Autodesk Inventor part; units mm, degrees
ref_plane "YZ Plane" through (0, 0, 0) normal (1, 0, 0) x (0, 1, 0)
ref_plane "XZ Plane" through (0, 0, 0) normal (0, 1, 0) x (-1, 0, 0)
ref_plane "XY Plane" through (0, 0, 0) normal (0, 0, 1) x (1, 0, 0)
sketch "Sketch1" plane through (0, 0, 0) normal (0, 0, 1) x (1, 0, 0)
  line L0 (-22.529, 12.5) -> (-14.529, 12.5)
  line L1 (22.5896, 12.5) -> (14.571, 12.5)
  line L2 (12.171, 14.9) -> (22.5896, 14.9)
  line L3 (22.5896, 14.9) -> (22.5896, 12.5)
  line L4 (-12.129, 14.9) -> (-22.529, 14.9)
  line L5 (-22.529, 14.9) -> (-22.529, 12.5)
  line L6 (-12.129, 0) -> (-12.129, 14.9)
  line L7 (12.171, 0) -> (12.171, 14.9)
  arc A0 (-12.129, 0) -> (12.171, 0) centre (0.021, 0) ccw
  arc A1 (-14.529, 0) -> (14.571, 0) centre (0.021, 0) ccw
  line L8 (-14.529, 12.5) -> (-14.529, -0.0004)
  line L9 (14.571, 12.5) -> (14.571, 0)
  point P0 (0, 0)
  point P1 (14.6524, 0.7379)
  dimension "d34" = 14.9
  dimension "d35" = 14.9
  dimension "d38" = 2.4
  dimension "d39" = 2.4
  dimension "d46" = 24.3
  dimension "d47" = 2.4
  dimension "d48" = 2.4
extrude "Extrusion5" add sketch "Sketch1" along normal blind 6
fillet "Fillet7" radius 1 1 edges at (14.571, 12.5, 3)
fillet "Fillet8" radius 1 1 edges at (-14.529, 12.5, 3)
sketch "Sketch5" plane through (12.171, 14.9, 0) normal (0, 1, 0) x (1, 0, 0)
  line L0 (10.4185, 0) -> (10.4185, -6)
  line L1 (3.4, 0) -> (10.4185, 0)
  circle A0 centre (5.2093, -3) radius 1.5
  circle A1 centre (-29.5299, -3.1217) radius 1.5
  point P0 (-12.171, 0)
  dimension "d54" = 3
extrude "Extrusion6" cut sketch "Sketch5" against normal blind 10
properties part number "motor_support_v2" material "PET Plastic"
For this review, take the finished solid that the model builds, in its own axes (mm). A direction names the side the tool comes from. Give positions to 0.01 mm unless a question says otherwise; leave off trailing zeros. Loops run counter-clockwise (first coordinate to the right, second up) from the corner with the lowest first, then second, coordinate; pieces in that order, holes last. Notation, with made-up numbers: M 12,56.25 L 44,56.25 A28 ccw 44,78.25 Z; hole C -26,-31.75 d4. An arc over 180 degrees is marked long. Answer as a JSON object with one key per item and string values. Group by question number.
Q1. Add section C-C on y = 7. Give the boundary of the cut face in (x, z), and give its area (3 significant figures).
Q2. Add section A-A on y = -9.75. Give the boundary of the cut face in (x, z).
Q3. Mouldability with a two-part tool opening along X and no side actions: class faces 1 (the flat face through (22.59, 14, 3)), 2 (the flat face through (-12, -3, 0)), 3 (the flat face through (12.171, 7, 3)), 4 (the flat face through (-12.129, 7, 3)) as +X half, -X half, draft (parallel to the pull), parting line (faces both ways), or undercut.
Q4. Insertion check: P1, Ø3, axis at y = 4.5, z = 4, coming from the +X side; P2, Ø2.5, axis at x = -17.36, z = 3.12, coming from the +Y side; P3, Ø1.8, axis at x = -19.5, z = 3, coming from the -Y side; P4, Ø3, axis at y = 5, z = 4, coming from the -X side. Each pin has a flat end and moves straight along its axis. Give the tip position at first contact, or say it passes through.
Q5. Tool access review of faces 5 (the flat face through (-19.1, 12.5, 3)), 6 (the flat face through (16, 14.9, 2)), 7 (the flat face through (19.1, 12.5, 3)): name each direction out of +Z, -Z, +X, -X, +Y, -Y from which nothing blocks a thin tool from reaching the whole face with its end or side.
Q6. Add section D-D on x = -4. Give the boundary of the cut face in (y, z).
Q7. Add section B-B on z = 2.45. Give the boundary of the cut face in (x, y), and give its area (3 significant figures).
Q8. For probe 1 along X at (y, z) = (13.55, 3); probe 2 along X at (y, z) = (3.5, 4.4); probe 3 along Y at (x, z) = (17, 4.65), list the stretches that pass through material, from the lowest coordinate up. Write a range as [from, to].
Checked values:
{
 "1": {"outline": "M -14.53,0 L -12.13,0 L -12.13,6 L -14.53,6 Z; M 12.17,0 L 14.57,0 L 14.57,6 L 12.17,6 Z", "area": "28.8 mm²"},
 "2": {"outline": "M -10.78,0 L -7.23,0 L -7.23,6 L -10.78,6 Z; M 7.27,0 L 10.82,0 L 10.82,6 L 7.27,6 Z"},
 "3": {"face 1": "+X half", "face 2": "draft", "face 3": "undercut", "face 4": "undercut"},
 "4": {"P1": "x = 14.57", "P2": "through", "P3": "y = 12.5", "P4": "x = -14.53"},
 "5": {"face 5": "+Z, -Z, -X, -Y", "face 6": "+Z, -Z, +X, -X, +Y", "face 7": "+Z, -Z, +X, -Y"},
 "6": {"outline": "M -13.98,0 L -11.47,0 L -11.47,6 L -13.98,6 Z"},
 "7": {"outline": "M -22.53,12.5 L -18.7,12.5 L -18.7,14.9 L -22.53,14.9 Z; M -16.02,12.5 L -15.53,12.5 A1 cw -14.53,11.5 L -14.53,0 A14.55 ccw 14.57,0 L 14.57,11.5 A1 cw 15.57,12.5 L 15.98,12.5 L 15.98,14.9 L 12.17,14.9 L 12.17,0 A12.15 cw -12.13,0 L -12.13,14.9 L -16.02,14.9 Z; M 18.78,12.5 L 22.59,12.5 L 22.59,14.9 L 18.78,14.9 Z", "area": "198 mm²"},
 "8": {"probe 1": "[-22.53, -18.85], [-15.86, -12.13], [12.17, 15.88], [18.88, 22.59]", "probe 2": "[-14.53, -12.13], [12.17, 14.57]", "probe 3": "[12.5, 14.9]"}
}
